For this review, take the finished solid that the model builds, in its own axes (mm). Face numbers are marked on the shaded views. A direction names the side the tool comes from. Coordinates: 2 decimals unless noted, no trailing zeros. Order: outer loops, then holes, each group sorted by start corner. A loop starts at its lowest first (then second) coordinate and runs counter-clockwise, first axis right, second up. Notation, with made-up numbers: (19, -18.5) -> (32, -18.5) arc R18 cw to (32, 4.5) -> close; hole circle Ø4 at (48, 51). An arc over 180 degrees is marked (long way). Return JSON: item names as keys, results as strings. Group by question number.
Item 1: Take a section at A-A (y = 23.5). Write out the cut boundary in (x, z).
Item 2: Insertion check: pin 1 (6 mm diameter, centred on y = 16.5, z = -7, fed in from +X); pin 2 (2 mm diameter, centred on y = 22, z = 4.5, fed in from -X); pin 3 (6 mm diameter, centred on x = -6, y = 7, fed in from -Z). Each pin has a flat end and moves straight along its axis. Give the tip position at first contact, or say it passes through.
Item 3: Machinability: for the marked faces 4 and 5, which of the approach directions +Z, -Z, +X, -X, +Y, -Y give a long, thin tool a straight path to every point of the face, cutting with its end or side? Answer none if there is none.
Item 4: Take a section at B-B (x = -4.5). Count the separate pieces of the cut face and the enclosed holes in it, then the cut area to 3 significant figures.
Item 5: For line 1 along Y through (x, z) = (0, -5.25); line 2 along Y through (x, z) = (-8, 4); line 3 along Z through (x, y) = (0, 11.75), list the stretches that pass through material, from the lowest coordinate up.
Item 6: Draft analysis for pull direction Z (two halves, no side actions). For the marked faces 1, 2 and 3, state which applies: +Z half, -Z half, draft (parallel to the pull), parting line (faces both ways), or undercut.
Autodesk Inventor part; units mm, degrees
ref_plane "Work Plane1" through (0, 25, -10) normal (0, 0, -1) x (-1, 0, 0)
ref_plane "Work Plane3" through (-9.6593, 25, 2.5882) normal (-0.9659, 0, 0.2588) x (0, -1, 0)
ref_plane "YZ Plane" through (0, 0, 0) normal (1, 0, 0) x (0, 1, 0)
sketch "Sketch1" plane through (0, 0, 0) normal (0, 1, 0) x (-1, 0, 0)
  circle A0 centre (0, 0) radius 10
  dimension "d0" = 20
extrude "Extrusion1" add sketch "Sketch1" along normal blind 25
sketch "Sketch2" plane through (0, 25, 0) normal (0, 1, 0) x (1, 0, 0)
  circle A0 centre (0, 0) radius 10
  circle A1 centre (0, 0) radius 2.5
  dimension "d3" = 5
extrude "Extrusion2" cut sketch "Sketch2" against normal blind 14 contours A1
sketch "Sketch3" plane through (0, 0, 0) normal (0, -1, 0) x (1, 0, 0)
  circle A0 centre (0, 0) radius 10
  circle A1 centre (0, 0) radius 2.5
  dimension "d6" = 5
extrude "Extrusion3" cut sketch "Sketch3" against normal blind 11 contours A1
chamfer "Chamfer1" distance 1 angle 45 2 edges at (10, 25, 0) (10, 0, 0)
chamfer "Chamfer2" distance 0.5 angle 45 2 edges at (-2.5, 25, 0) (-2.5, 0, 0)
sketch "Sketch4" plane through (0, 25, 0) normal (0, 1, 0) x (1, 0, 0)
  circle A0 centre (0, 0) radius 9
  circle A1 centre (0, 0) radius 3
  circle A2 centre (0, 0) radius 10
  line L0 (-10, 0) -> (10, 0) construction
  line L1 (0, 0) -> (-9.6593, -2.5882) construction
  point P0 (0, 10)
  point P1 (-9.6593, -2.5882)
  dimension "d28" = 15
ref_plane "Work Plane1" through (0, 25, -10) normal (0, 0, -1) x (-1, 0, 0)
ref_plane "Work Plane3" through (-9.6593, 25, 2.5882) normal (-0.9659, 0, 0.2588) x (0, -1, 0)
sketch "Sketch5" plane through (0, 25, -10) normal (0, 0, -1) x (-1, 0, 0)
  line L0 (10, -1) -> (-10, -1)
  line L1 (-10, -24) -> (10, -24)
  line L2 (-10, -24) -> (-10, -1)
  line L3 (10, -24) -> (10, -1)
  circle A0 centre (0, -4.5) radius 2
  circle A1 centre (0, -20.5) radius 2
  line L4 (-9, 0) -> (9, 0)
  line L5 (9, -25) -> (-9, -25)
  point P0 (0, -25)
  point P1 (0, -1)
  dimension "d16" = 4
  dimension "d17" = 4
  dimension "d18" = 4.5
  dimension "d19" = 4.5
extrude "Extrusion4" cut sketch "Sketch5" against normal blind 8.75 contours A0 | A1
sketch "Sketch6" plane through (-9.6593, 25, 2.5882) normal (-0.9659, 0, 0.2588) x (0, -1, 0)
  circle A0 centre (4.5, 0) radius 2
  line L0 (24, -10) -> (1, -10)
  line L1 (24, 10) -> (1, 10)
  line L2 (25, 9) -> (25, -9)
  line L3 (0, -9) -> (0, 9)
  circle A1 centre (20.5, 0) radius 2
  point P0 (25, 0)
  point P1 (0, 0)
  dimension "d22" = 4
  dimension "d23" = 4
  dimension "d24" = 4.5
  dimension "d25" = 4.5
extrude "Extrusion5" cut sketch "Sketch6" against normal blind 8.75
thread "Thread1"
thread "Thread2"
thread "Thread3"
thread "Thread4"
properties part number "ZACMEFlexCoupler" material "Aluminum 6061"
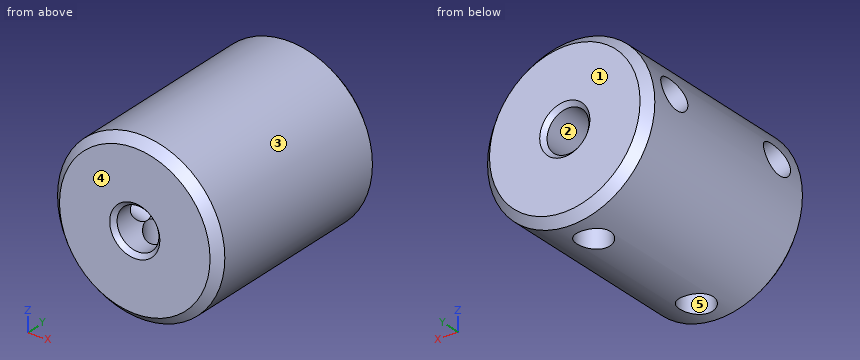
Findings below:
{
 "1": {"outline": "circle Ø20 at (0, 0); hole circle Ø5 at (0, 0)"},
 "2": {"pin 1": "stops at x = 9.17", "pin 2": "stops at x = -9.36", "pin 3": "stops at z = -9.54"},
 "3": {"face 4": "+Z, -Z, +X, -X, -Y", "face 5": "-Z"},
 "4": {"separate pieces": "1", "enclosed holes": "2", "area": "418 mm2"},
 "5": {"line 1": "y = 0 to 2.5, 6.5 to 18.5, 22.5 to 25", "line 2": "y = 0 to 3.61, 5.39 to 19.61, 21.39 to 25", "line 3": "z = -10 to -2.5, 2.5 to 10"},
 "6": {"face 1": "draft", "face 2": "undercut", "face 3": "parting line"}
}
